Can you work these out from the model? Positions are in its coordinate system, mm. A direction names the side the tool comes from. Round coordinates to 2 decimals unless told otherwise and drop trailing zeros. Loops run counter-clockwise (first coordinate to the right, second up) from the corner with the lowest first, then second, coordinate; pieces in that order, holes last. Notation, with made-up numbers: (33.5, -29.5) -> (53.5, -29.5) arc R38 ccw to (53.5, 8.5) -> close; hole circle Ø9 at (-12, 32.25). An arc over 180 degrees is marked (long way). Use a Markdown table: item, result.
from build123d import *

# Parameters (mm, degrees)
SKETCH1_R           = 14
BOSS_EXTRUDE1_DEPTH = 8
SKETCH2_W           = 40
SKETCH2_H           = 8
BOSS_EXTRUDE2_DEPTH = 20
SKETCH3_R           = 2.65
CUT_EXTRUDE1_DEPTH  = 37.5
FILLET1_R           = 2


with BuildPart() as part:
    # Sketch1 → Boss-Extrude1 (new body)
    with BuildSketch(Plane.XY):
        with BuildLine():
            Line((-20, 0), (-20, -71.5))
            Line((-20, -71.5), (20, -71.5))
            Line((20, -71.5), (20, 0))
            ThreePointArc((20, 0), (0, 20), (-20, 0))
        make_face()
        Circle(SKETCH1_R, mode=Mode.SUBTRACT)
    extrude(amount=BOSS_EXTRUDE1_DEPTH)

    # Sketch2 → Boss-Extrude2 (add)
    with BuildSketch(Plane.XY.offset(8)):
        with Locations((0, -39)):
            Rectangle(SKETCH2_W, SKETCH2_H)
        with Locations((0, -67.5)):
            Rectangle(SKETCH2_W, SKETCH2_H)
    extrude(amount=BOSS_EXTRUDE2_DEPTH)

    # Sketch3 → Cut-Extrude1 (cut, through all)
    with BuildSketch(Plane(origin=(0, -35, 0), x_dir=(1, 0, 0), z_dir=(0, 1, 0))):
        with Locations((-12.5, -18)):
            Circle(SKETCH3_R)
        with Locations((12.5, -18)):
            Circle(SKETCH3_R)
    extrude(amount=-CUT_EXTRUDE1_DEPTH, mode=Mode.SUBTRACT)

    # Fillet1
    fillet1_edges = [part.edges().sort_by_distance(p)[0] for p in [
        (20, -17.5, 8),
        (-20, -35, 18),
        (0, -35, 8),
        (20, -35, 18),
        (-20, -39, 28),
        (20, -39, 28),
        (0, -35, 28),
        (20, -67.5, 28),
        (-20, -67.5, 28),
        (0, -71.5, 28),
        (0, 20, 8),
        (0, -71.5, 0),
        (20, -71.5, 14),
        (-20, -71.5, 14),
        (-20, -17.5, 8),
    ]]
    fillet(fillet1_edges, radius=FILLET1_R)


solid = part.part
1. I want a section at A-A (y = -41.5). Please give me the cut outline in (x, z), plus the area to 3 significant figures.
Answer sheet:
| item | result |
|---|---|
| outline | (-20, 0) -> (20, 0) -> (20, 26) arc R2 ccw to (18, 28) -> (-18, 28) arc R2 ccw to (-20, 26) -> close; hole circle Ø5.3 at (-12.5, 18); hole circle Ø5.3 at (12.5, 18) |
| area | 1,070 mm² |
2. Which directions (+Z, -Z, +X, -X, +Y, -Y) give clear straight access to the entire face, cutting with the end or side of a thin tool? Please do faces 1 (the cylindrical face through (19.4, -16.27, 7.43)), 2 (the cylindrical face through (-19.43, -35.6, 18.11)), 3 (the flat face through (0, -53, 8)).
Answer sheet:
| item | result |
|---|---|
| face 1 | +Z, +X, +Y |
| face 2 | +Z, -X, +Y |
| face 3 | +Z, +X, -X |
3. If we mould it in two halves opening along X, with no side actions, what happens to faces 4 (the cylindrical face through (-10.05, -67.44, 19.01)), 5 (the cylindrical face through (-19.43, -39.96, 27.4)), 6 (the cylindrical face through (0, 20, 3)), 7 (the cylindrical face through (14.95, -67.44, 19.01))? For each: +X half, -X half, draft (parallel to the pull), parting line (faces both ways), or undercut.
Answer sheet:
| item | result |
|---|---|
| face 4 | undercut |
| face 5 | -X half |
| face 6 | parting line |
| face 7 | undercut |
4. I want a section at B-B (z = 25). Please give me the cut outline in (x, y), plus the area to 3 significant figures.
Answer sheet:
| item | result |
|---|---|
| outline | (-20, -69.5) arc R2 ccw to (-18, -71.5) -> (18, -71.5) arc R2 ccw to (20, -69.5) -> (20, -63.5) -> (-20, -63.5) -> close; (-20, -43) -> (20, -43) -> (20, -37) arc R2 ccw to (18, -35) -> (-18, -35) arc R2 ccw to (-20, -37) -> close |
| area | 637 mm² |
5. I want a section at C-C (x = 0). Please give me the cut outline in (y, z).
Answer sheet:
| item | result |
|---|---|
| outline | (-71.5, 2) arc R2 ccw to (-69.5, 0) -> (-14, 0) -> (-14, 8) -> (-33, 8) arc R2 cw to (-35, 10) -> (-35, 26) arc R2 ccw to (-37, 28) -> (-43, 28) -> (-43, 8) -> (-63.5, 8) -> (-63.5, 28) -> (-69.5, 28) arc R2 ccw to (-71.5, 26) -> close; (14, 0) -> (20, 0) -> (20, 6) arc R2 ccw to (18, 8) -> (14, 8) -> close |
6. I want a section at D-D (y = -2). Please give me the cut outline in (x, z).
Answer sheet:
| item | result |
|---|---|
| outline | (-20, 0) -> (-13.86, 0) -> (-13.86, 8) -> (-18, 8) arc R2 ccw to (-20, 6) -> close; (13.86, 0) -> (20, 0) -> (20, 6) arc R2 ccw to (18, 8) -> (13.86, 8) -> close |
7. Will these pins go through, and if not, where does the flat tip stop? pin 1 Ø6 at (x, z) = (4, 15.5) entering from +Y; pin 2 Ø10 at (x, y) = (-10, -51.5) entering from +Z.
Answer sheet:
| item | result |
|---|---|
| pin 1 | stops at y = -35 |
| pin 2 | stops at z = 8 |
8. I need wall thicknesses on line 1 (X direction, y = -40.75, z = 18); line 2 (Y direction, x = 2, z = 17); line 3 (X direction, y = -40, z = 15.75). Which ranges of each line are inside material? Lowest first, please.
Answer sheet:
| item | result |
|---|---|
| line 1 | x = -20 to -15.15, -9.85 to 9.85, 15.15 to 20 |
| line 2 | y = -71.5 to -63.5, -43 to -35 |
| line 3 | x = -20 to -13.9, -11.1 to 11.1, 13.9 to 20 |
